Answer from the drawing. Dimensions are ordinates in mm from the lowest x, y and z of the part. A direction names the side the tool comes from. Round coordinates to 2 decimals unless told otherwise and drop trailing zeros. Loops run counter-clockwise (first coordinate to the right, second up) from the corner with the lowest first, then second, coordinate; pieces in that order, holes last. Notation, with made-up numbers: M -17.75,66.5 L -5.75,66.5 A14 cw -5.75,84.5 Z; hole C 62.25,40.5 d1. An arc over 180 degrees is marked long. Answer as a JSON object with one key per item and string values.
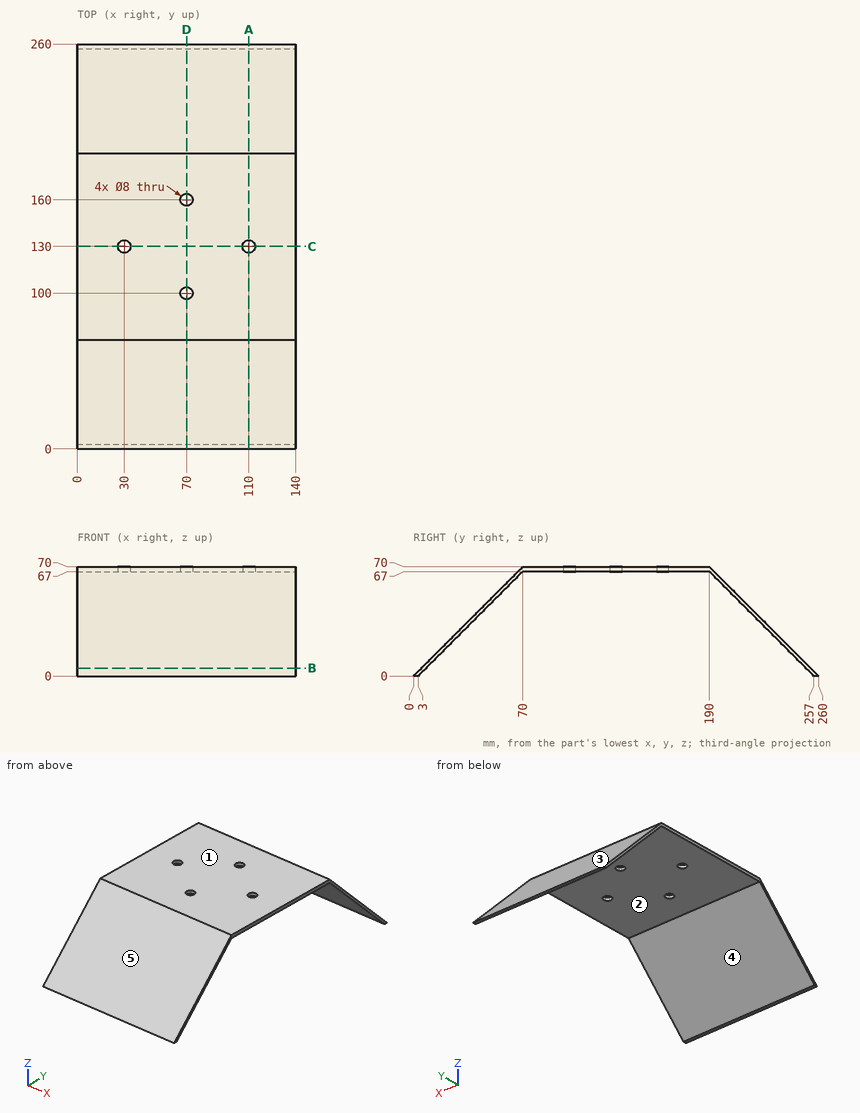
Item 1: The part is cut by section D-D (x = 70). Give the vertices of the cut face in (y, z), then the cut area to 3 significant figures.
Values follow:
{"outline": "M 0,0 L 3,0 L 70,67 L 96,67 L 96,70 L 70,70 Z; M 104,67 L 156,67 L 156,70 L 104,70 Z; M 164,67 L 190,67 L 257,0 L 260,0 L 190,70 L 164,70 Z", "area": "723 mm^2"}
Item 2: Flat-ended cylindrical pins translate along their axes: P1, Ø13, axis at x = 70, y = 160, coming from the -Z side; P2, Ø3, axis at x = 31, z = 31.5, coming from the +Y side; P3, Ø1.5, axis at x = 43, z = 10.5, coming from the -Y side. Find the tip coordinate at first contact, or state that the pin passes through.
Values follow:
{"P1": "z = 67", "P2": "y = 230", "P3": "y = 9.75"}
Item 3: The part is cut by section B-B (z = 5). Give the vertices of the cut face in (x, y), then the cut area to 3 significant figures.
Values follow:
{"outline": "M 0,5 L 140,5 L 140,8 L 0,8 Z; M 0,252 L 140,252 L 140,255 L 0,255 Z", "area": "840 mm^2"}
Item 4: Straight lines are drawn through the part: line 1 (X direction, y = 130, z = 69); line 2 (X direction, y = 100, z = 67.85); line 3 (Z direction, x = 32, y = 112). For each, find the intervals that lie inside material, in ascending order.
Values follow:
{"line 1": "0 to 26, 34 to 106, 114 to 140", "line 2": "0 to 66, 74 to 140", "line 3": "67 to 70"}
Item 5: The part is cut by section C-C (y = 130). Give the vertices of the cut face in (x, z), then the cut area to 3 significant figures.
Values follow:
{"outline": "M 0,67 L 26,67 L 26,70 L 0,70 Z; M 34,67 L 106,67 L 106,70 L 34,70 Z; M 114,67 L 140,67 L 140,70 L 114,70 Z", "area": "372 mm^2"}
Item 6: Determine the mould class of the marked faces 3, 4 and 5 for opening direction Y: released by +Y, released by -Y, zero draft, split by the parting line, or undercut.
Values follow:
{"face 3": "released by +Y", "face 4": "undercut", "face 5": "released by -Y"}
Item 7: Which of the six approach directions +Z, -Z, +X, -X, +Y, -Y give full straight-line access (tool end or side, diameter ignored) to the marked faces 1 and 2?
Values follow:
{"face 1": "+Z, +X, -X, +Y, -Y", "face 2": "-Z, +X, -X"}
Item 8: The part is cut by section A-A (x = 110). Give the vertices of the cut face in (y, z), then the cut area to 3 significant figures.
Values follow:
{"outline": "M 0,0 L 3,0 L 70,67 L 126,67 L 126,70 L 70,70 Z; M 134,67 L 190,67 L 257,0 L 260,0 L 190,70 L 134,70 Z", "area": "747 mm^2"}
